The model under review builds one solid part; all positions refer to its coordinate system, in mm. A direction names the side the tool comes from. Coordinates: 2 decimals unless noted, no trailing zeros. Write each loop counter-clockwise with the first axis right and the second up, starting at its lowest first coordinate (ties: lowest second). Pieces come first, ordered by that corner, then holes.
1) Add section C-C, the plane y = -2.25. State the section outline as (x, z) points (3 decimals), then the cut area to 3 significant figures.
2) For P1, Ø3, axis at x = -16.5, z = 0, coming from the -Y side; P2, Ø1, axis at x = 8, z = 14.5, coming from the +Y side; P3, Ø4, axis at y = -2.5, z = 17, coming from the -X side; P4, Ø1, axis at x = 7.5, y = 0.5, coming from the -Z side, all flat-tipped, find the tip position at first contact; note any pin that passes through.
3) Machinability: for faces 1 (the cylindrical face through (0.07, 4.51, -20)), 2 (the flat face through (-1, 4, 17)), 3 (the cylindrical face through (-9.09, 3.03, 13.75)), which of the approach directions +Z, -Z, +X, -X, +Y, -Y give a long, thin tool a straight path to every point of the face, cutting with its end or side? Answer none if there is none.
4) Add section A-A, the plane x = 0. Give the number of separate pieces and of enclosed holes in the cut face, then the cut area to 3 significant figures.
5) For line 1 (X direction, y = -1.5, z = 0) (3 decimals); line 2 (X direction, y = 2.2, z = 0); line 3 (Y direction, x = 18, z = 0), list the stretches that pass through material, from the lowest coordinate up.
6) Mouldability with a two-part tool opening along X and no side actions: class faces 4 (the flat face through (10, 5, 0)), 5 (the cylindrical face through (-12.93, 2.465, -16.863)), 6 (the flat face through (8, 1, -14)), 7 (the flat face through (-8, 1, -14)) as released by +X, released by -X, zero draft, split by the parting line, or undercut.
7) Add section B-B, the plane z = -17.5. State the section outline as (x, y) points, then the cut area to 3 significant figures.
from build123d import *

# Parameters (mm, degrees)
SKETCH1_R           = 21.25
BOSS_EXTRUDE1_DEPTH = 5
SKETCH2_R           = 1.5
CUT_EXTRUDE1_DEPTH  = 5
SKETCH3_R           = 2
CUT_EXTRUDE2_DEPTH  = 4
CIRPATTERN1_COUNT   = 2
SKETCH5_R           = 14
BOSS_EXTRUDE2_DEPTH = 0.25
SKETCH6_R           = 12.575
BOSS_EXTRUDE3_DEPTH = 4
CHAMFER1_SIZE       = 0.5
SKETCH7_R           = 9.5
CUT_EXTRUDE3_DEPTH  = 9.25
SKETCH8_R           = 1
CUT_EXTRUDE4_DEPTH  = 4
CIRPATTERN2_COUNT   = 6


with BuildPart() as part:
    # Sketch1 → Boss-Extrude1 (new body)
    with BuildSketch(Plane(origin=(0, 0, 0), x_dir=(1, 0, 0), z_dir=(0, 1, 0))):
        with Locations(Location((0, 0, 0), (0, 0, 270))):
            Circle(SKETCH1_R)
    extrude(amount=BOSS_EXTRUDE1_DEPTH)

    # Sketch2 → Cut-Extrude1 (cut)
    with BuildSketch(Plane(origin=(0, 5, 0), x_dir=(1, 0, 0), z_dir=(0, 1, 0))):
        with Locations(Location((0, 18.5, 0), (0, 0, 270))):
            Circle(SKETCH2_R)
    cut_extrude1 = extrude(amount=-CUT_EXTRUDE1_DEPTH, mode=Mode.SUBTRACT)

    # Sketch3 → Cut-Extrude2 (cut)
    with BuildSketch(Plane.XZ):
        with Locations(Location((0, -18.5, 0), (0, 0, 270))):
            Circle(SKETCH3_R)
    cut_extrude2 = extrude(amount=-CUT_EXTRUDE2_DEPTH, mode=Mode.SUBTRACT)

    # CirPattern1: Cut-Extrude1, Cut-Extrude2 ×2 about axis
    cirpattern1_axis = Axis((0, 0, 0), (0, 1, 0))
    add([cut_extrude1.rotate(cirpattern1_axis, i * 360 / CIRPATTERN1_COUNT) for i in range(1, CIRPATTERN1_COUNT)], mode=Mode.SUBTRACT)
    add([cut_extrude2.rotate(cirpattern1_axis, i * 360 / CIRPATTERN1_COUNT) for i in range(1, CIRPATTERN1_COUNT)], mode=Mode.SUBTRACT)

    # Sketch5 → Boss-Extrude2 (add)
    with BuildSketch(Plane.XZ):
        with Locations(Location((0, 0, 0), (0, 0, 270))):
            Circle(SKETCH5_R)
    extrude(amount=BOSS_EXTRUDE2_DEPTH)

    # Sketch6 → Boss-Extrude3 (add)
    with BuildSketch(Plane.XZ.offset(0.25)):
        with Locations(Location((0, 0, 0), (0, 0, 270))):
            Circle(SKETCH6_R)
    extrude(amount=BOSS_EXTRUDE3_DEPTH)

    # Chamfer1
    chamfer1_edges = [part.edges().sort_by_distance(p)[0] for p in [
        (0, -4.25, 12.575),
    ]]
    chamfer(chamfer1_edges, length=CHAMFER1_SIZE)

    # Sketch7 → Cut-Extrude3 (cut)
    with BuildSketch(Plane.XZ.offset(4.25)):
        with Locations(Location((0, 0, 0), (0, 0, 270))):
            Circle(SKETCH7_R)
    extrude(amount=-CUT_EXTRUDE3_DEPTH, mode=Mode.SUBTRACT)

    # Sketch8 → Cut-Extrude4 (cut)
    with BuildSketch(Plane(origin=(0, 5, 0), x_dir=(1, 0, 0), z_dir=(0, 1, 0))):
        with Locations(Location((8.25, 14.289419162, 0), (0, 0, 270))):
            Circle(SKETCH8_R)
    cut_extrude4 = extrude(amount=-CUT_EXTRUDE4_DEPTH, mode=Mode.SUBTRACT)

    # CirPattern2: Cut-Extrude4 ×6 about axis
    cirpattern2_axis = Axis((0, 0, 0), (0, 1, 0))
    for i in range(1, CIRPATTERN2_COUNT):
        add(cut_extrude4.rotate(cirpattern2_axis, i * 360 / CIRPATTERN2_COUNT), mode=Mode.SUBTRACT)


solid = part.part
Geometry results:
1. outline: circle Ø25.15 at (0, 0); hole circle Ø19 at (0, 0)
1. area: 213 mm2
2. P1: stops at y = 0
2. P2: stops at y = 1
2. P3: passes through
2. P4: stops at z = -20.06
3. face 1: +Y, -Y
3. face 2: -Y
3. face 3: +Y
4. separate pieces: 4
4. enclosed holes: 0
4. area: 106 mm2
5. line 1: x = -12.575 to -9.5, 9.5 to 12.575
5. line 2: x = -21.25 to -17.5, -15.5 to -9.5, 9.5 to 15.5, 17.5 to 21.25
5. line 3: y = 0 to 5
6. face 4: zero draft
6. face 5: split by the parting line
6. face 6: undercut
6. face 7: undercut
7. outline: (-12.05, 0) - (-1.73, 0) - (-1.73, 4) - (-1.12, 4) - (-1.12, 5) - (-12.05, 5) - close; (1.12, 4) - (1.73, 4) - (1.73, 0) - (12.05, 0) - (12.05, 5) - (1.12, 5) - close
7. area: 104 mm2
